```python
from build123d import *

# Parameters (mm, degrees)
SKETCH1_W           = 17
SKETCH1_H           = 4.25
BOSS_EXTRUDE1_DEPTH = 2.9
SKETCH2_W           = 15.4
SKETCH2_H           = 1.9
CUT_EXTRUDE1_DEPTH  = 2.9
SKETCH3_W           = 0.3
SKETCH3_H           = 0.6
BOSS_EXTRUDE2_DEPTH = 2.5
SKETCH4_W           = 0.3
SKETCH4_H           = 0.8
BOSS_EXTRUDE3_DEPTH = 0.3


with BuildPart() as part:
    # Sketch1 → Boss-Extrude1 (new body)
    with BuildSketch(Plane.XY):
        Rectangle(SKETCH1_W, SKETCH1_H)
    extrude(amount=BOSS_EXTRUDE1_DEPTH)

    # Sketch2 → Cut-Extrude1 (cut)
    with BuildSketch(Plane.XZ.offset(2.125)):
        with Locations((0, 1.45)):
            Rectangle(SKETCH2_W, SKETCH2_H)
    extrude(amount=-CUT_EXTRUDE1_DEPTH, mode=Mode.SUBTRACT)

    # Sketch3 → Boss-Extrude2 (add)
    with BuildSketch(Plane.XZ.offset(-0.775)):
        with Locations((-7, 1.45)):
            Rectangle(SKETCH3_W, SKETCH3_H)
        with Locations((-6, 1.45)):
            Rectangle(SKETCH3_W, SKETCH3_H)
        with Locations((-5, 1.45)):
            Rectangle(SKETCH3_W, SKETCH3_H)
        with Locations((-4, 1.45)):
            Rectangle(SKETCH3_W, SKETCH3_H)
        with Locations((-3, 1.45)):
            Rectangle(SKETCH3_W, SKETCH3_H)
        with Locations((-2, 1.45)):
            Rectangle(SKETCH3_W, SKETCH3_H)
        with Locations((-1, 1.45)):
            Rectangle(SKETCH3_W, SKETCH3_H)
        with Locations((0, 1.45)):
            Rectangle(SKETCH3_W, SKETCH3_H)
        with Locations((1, 1.45)):
            Rectangle(SKETCH3_W, SKETCH3_H)
        with Locations((2, 1.45)):
            Rectangle(SKETCH3_W, SKETCH3_H)
        with Locations((3, 1.45)):
            Rectangle(SKETCH3_W, SKETCH3_H)
        with Locations((4, 1.45)):
            Rectangle(SKETCH3_W, SKETCH3_H)
        with Locations((5, 1.45)):
            Rectangle(SKETCH3_W, SKETCH3_H)
        with Locations((6, 1.45)):
            Rectangle(SKETCH3_W, SKETCH3_H)
        with Locations((7, 1.45)):
            Rectangle(SKETCH3_W, SKETCH3_H)
    extrude(amount=BOSS_EXTRUDE2_DEPTH)

    # Sketch4 → Boss-Extrude3 (add)
    with BuildSketch(Plane(origin=(0, 0, 0), x_dir=(-1, 0, 0), z_dir=(0, 0, -1))):
        with Locations((-7, 2.425)):
            Rectangle(SKETCH4_W, SKETCH4_H)
        with Locations((-6, 2.425)):
            Rectangle(SKETCH4_W, SKETCH4_H)
        with Locations((-5, 2.425)):
            Rectangle(SKETCH4_W, SKETCH4_H)
        with Locations((-4, 2.425)):
            Rectangle(SKETCH4_W, SKETCH4_H)
        with Locations((-3, 2.425)):
            Rectangle(SKETCH4_W, SKETCH4_H)
        with Locations((-2, 2.425)):
            Rectangle(SKETCH4_W, SKETCH4_H)
        with Locations((-1, 2.425)):
            Rectangle(SKETCH4_W, SKETCH4_H)
        with Locations((0, 2.425)):
            Rectangle(SKETCH4_W, SKETCH4_H)
        with Locations((1, 2.425)):
            Rectangle(SKETCH4_W, SKETCH4_H)
        with Locations((2, 2.425)):
            Rectangle(SKETCH4_W, SKETCH4_H)
        with Locations((3, 2.425)):
            Rectangle(SKETCH4_W, SKETCH4_H)
        with Locations((4, 2.425)):
            Rectangle(SKETCH4_W, SKETCH4_H)
        with Locations((5, 2.425)):
            Rectangle(SKETCH4_W, SKETCH4_H)
        with Locations((6, 2.425)):
            Rectangle(SKETCH4_W, SKETCH4_H)
        with Locations((7, 2.425)):
            Rectangle(SKETCH4_W, SKETCH4_H)
    extrude(amount=-BOSS_EXTRUDE3_DEPTH)


solid = part.part
```
Design review of the part built by this model. Coordinates are the model's own, in mm. A direction names the side the tool comes from. Round coordinates to 2 decimals unless told otherwise and drop trailing zeros. Write each loop counter-clockwise with the first axis right and the second up, starting at its lowest first coordinate (ties: lowest second). Pieces come first, ordered by that corner, then holes.
Item 1: We need section B-B on y = -0.6. State how many separate pieces and enclosed holes the cut face has, and give its area (3 significant figures).
Item 2: We need section A-A on x = -4.5. Write out the cut boundary in (y, z) (3 decimals), and give its area (4 significant figures).
Item 3: The part is to be moulded in two halves that separate along Z. For faces 1 (the flat face through (0, 2.125, 1)), 2 (the flat face through (0, 0, 2.9)), 3 (the flat face through (0, 0, 0)), 4 (the flat face through (0, -1, 2.4)), say which applies: +Z half, -Z half, draft (parallel to the pull), parting line (faces both ways), or undercut.
Item 4: For faces 5 (the flat face through (0, -1, 0.5)), 6 (the flat face through (-8.5, 0, 1)), list the 3-axis set-ups (+Z, -Z, +X, -X, +Y, -Y) from which the entire face can be reached by the end or side of a thin tool; tool diameter is ignored.
Item 5: We need section C-C on z = 2.1. Write out the cut boundary in (x, y) (3 decimals), and give its area (3 significant figures).
Item 6: For probe 1 along Z at (x, y) = (-3.5, -1.25); probe 2 along Z at (x, y) = (-5, -0.9); probe 3 along X at (y, z) = (0.35, 0.55), list the stretches that pass through material, from the lowest coordinate up.
Returned:
1. separate pieces: 16
1. enclosed holes: 1
1. area: 22.7 mm2
2. outline: (-2.125, 0) - (2.125, 0) - (2.125, 2.9) - (-2.125, 2.9) - (-2.125, 2.4) - (0.775, 2.4) - (0.775, 0.5) - (-2.125, 0.5) - close
2. area: 6.815 mm2
3. face 1: draft
3. face 2: +Z half
3. face 3: -Z half
3. face 4: undercut
4. face 5: -Y
4. face 6: +Z, -Z, -X, +Y, -Y
5. outline: (-8.5, -2.125) - (-7.7, -2.125) - (-7.7, 0.775) - (7.7, 0.775) - (7.7, -2.125) - (8.5, -2.125) - (8.5, 2.125) - (-8.5, 2.125) - close
5. area: 27.6 mm2
6. probe 1: z = 0 to 0.5, 2.4 to 2.9
6. probe 2: z = 0 to 0.5, 1.15 to 1.75, 2.4 to 2.9
6. probe 3: x = -8.5 to -7.7, 7.7 to 8.5
